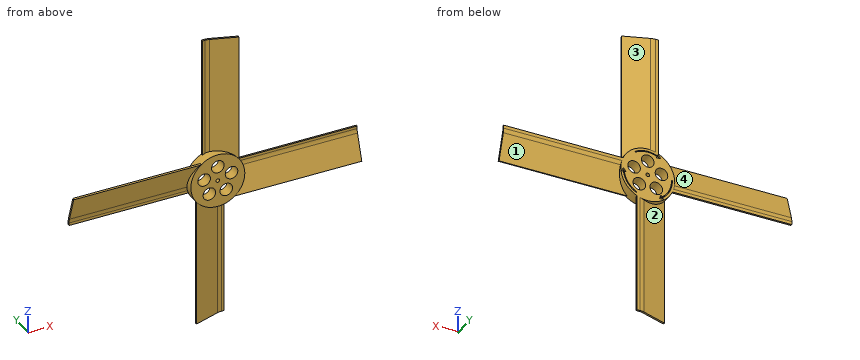
```python
from build123d import *

# Parameters (mm, degrees)
F1_DEPTH  = 80
F2_R      = 7.644408
F4_COUNT  = 4
F5_R      = 15
F6_DEPTH  = 6
F7_R      = 3.5
F7_R_2    = 1
F8_DEPTH  = 25
F10_DEPTH = 1


with BuildPart() as f1:
    # F0 (on Top) → F1 (new body)
    with BuildSketch(Plane.XY):
        Polygon((11.683772, -5.948683), (12, -5), (-3, 0), (-3.316228, -0.948683), align=None)
        Polygon((-3.316228, -0.948683), (-3, 0), (-6, 0), (-6, -0.948683), align=None)
    extrude(amount=-F1_DEPTH)

    # F2
    f2_edges = [f1.edges().sort_by_distance(p)[0] for p in [
        (-3.316228, -0.948683, -40),
        (-3, 0, -40),
    ]]
    fillet(f2_edges, radius=F2_R)



with BuildPart() as f4_1:
    # F4: instance of F1
    add(f1.part.rotate(Axis((0, 13.525062, 0), (0, 1, 0)), 1 * 360 / F4_COUNT))


with BuildPart() as f4_2:
    # F4: instance of F1
    add(f1.part.rotate(Axis((0, 13.525062, 0), (0, 1, 0)), 2 * 360 / F4_COUNT))


with BuildPart() as f4_3:
    # F4: instance of F1
    add(f1.part.rotate(Axis((0, 13.525062, 0), (0, 1, 0)), 3 * 360 / F4_COUNT))


with BuildPart() as f1_1:
    add(f1.part)

    add(f4_1.part)  # F6 merges F4_1

    add(f4_2.part)  # F6 merges F4_2

    add(f4_3.part)  # F6 merges F4_3
    # F5 (on Front) → F6 (join)
    with BuildSketch(Plane.XZ):
        Circle(F5_R)
    extrude(amount=F6_DEPTH)

    # F7 (on face) → F8 (cut)
    with BuildSketch(Plane(origin=(0, 0, 0), x_dir=(-1, 0, 0), z_dir=(0, 1, 0))):
        with Locations((-4.702282, 6.472136)):
            Circle(F7_R)
        with Locations((-7.608452, -2.472136)):
            Circle(F7_R)
        with Locations((0, -8)):
            Circle(F7_R)
        with Locations((7.608452, -2.472136)):
            Circle(F7_R)
        with Locations((4.702282, 6.472136)):
            Circle(F7_R)
        Circle(F7_R_2)
    extrude(amount=-F8_DEPTH, mode=Mode.SUBTRACT)

    # F9 (on face) → F10 (cut)
    with BuildSketch(Plane(origin=(0, 0, 0), x_dir=(-1, 0, 0), z_dir=(0, 1, 0))):
        with BuildLine():
            ThreePointArc((5.158171, -12.103592), (-1.067262, -13.113528), (-7.047458, -11.110221))
            Line((-7.047458, -11.110221), (-7.288358, -11.549476))
            ThreePointArc((-7.288358, -11.549476), (-1.091943, -13.613164), (5.354197, -12.563564))
            Line((5.354197, -12.563564), (5.746248, -13.483508))
            Line((5.746248, -13.483508), (7.096071, -11.549476))
            Line((7.096071, -11.549476), (4.76612, -11.183649))
            Line((4.76612, -11.183649), (5.158171, -12.103592))
        make_face()
        with BuildLine():
            Line((8.803936, 11.71815), (6.454104, 11.920116))
            Line((6.454104, 11.920116), (7.302264, 9.719405))
            Line((7.302264, 9.719405), (7.902933, 10.518903))
            ThreePointArc((7.902933, 10.518903), (11.89028, 5.632489), (13.145463, -0.548167))
            Line((13.145463, -0.548167), (13.646319, -0.537165))
            ThreePointArc((13.646319, -0.537165), (12.335317, 5.860932), (8.203267, 10.918652))
            Line((8.203267, 10.918652), (8.803936, 11.71815))
        make_face()
        with BuildLine():
            Line((-14.550184, 1.765357), (-13.550175, -0.370639))
            Line((-13.550175, -0.370639), (-12.068384, 1.464243))
            Line((-12.068384, 1.464243), (-13.061104, 1.584689))
            ThreePointArc((-13.061104, 1.584689), (-10.823018, 7.48104), (-6.098005, 11.658388))
            Line((-6.098005, 11.658388), (-6.357961, 12.086641))
            ThreePointArc((-6.357961, 12.086641), (-11.243374, 7.752232), (-13.557464, 1.644912))
            Line((-13.557464, 1.644912), (-14.550184, 1.765357))
        make_face()
    extrude(amount=-F10_DEPTH, mode=Mode.SUBTRACT)


with BuildPart() as f11_1:
    # F11: instance of F1
    add(f1_1.part.mirror(Plane.XY))


solid = f11_1.part
```
Check sheet for the modelled part. Datum: model origin and axes. Units: mm. Face numbers are marked on the shaded views. A direction names the side the tool comes from. Give positions to 0.01 mm unless a question says otherwise; leave off trailing zeros. Write each loop counter-clockwise with the first axis right and the second up, starting at its lowest first coordinate (ties: lowest second). Pieces come first, ordered by that corner, then holes.
Item 1: Cross-section at C-C (y = -3.5). Enter the section's corners in (x, z), and give its area (3 significant figures).
Item 2: Gauge pin test, flat ends, axial feed: pin 1 (6.5 mm diameter, centred on x = 7.61, z = 2.47, fed in from -Y); pin 2 (0.8 mm diameter, centred on x = 54, y = -0.5, fed in from +Z); pin 3 (0.5 mm diameter, centred on x = -40, y = -0.5, fed in from -Z); pin 4 (10 mm diameter, centred on x = 10.5, z = 18.5, fed in from +Y). Record the tip position at first contact, or that the pin passes through.
Item 3: Access from +Z, -Z, +X, -X, +Y, -Y to the whole of each face (thin tool, end or side, straight path). Record for the marked faces 1, 2, 3 and 4.
Item 4: Scan lines: L1, parallel to Z at x = 0, y = -1.9; L2, parallel to Z at x = 0, y = -3.9; L3, parallel to X at y = -2.5, z = 8.5. Record each from-to range of solid material in increasing order.
Item 5: Cross-section at B-B (x = -22.5). Enter the section's corners in (y, z), and give its area (3 significant figures).
Item 6: Cross-section at A-A (z = 57). Enter the section's corners in (x, y), and give its area (3 significant figures).
Report:
1. outline: (-80, 4.34) - (-14.36, 4.34) arc R15 ccw to (-7.5, -12.99) - (-7.5, -80) - (-4.34, -80) - (-4.34, -14.36) arc R15 ccw to (12.99, -7.5) - (80, -7.5) - (80, -4.34) - (14.36, -4.34) arc R15 ccw to (7.5, 12.99) - (7.5, 80) - (4.34, 80) - (4.34, 14.36) arc R15 ccw to (-12.99, 7.5) - (-80, 7.5) - close; hole circle Ø7 at (-7.61, 2.47); hole circle Ø7 at (-4.7, -6.47); hole circle Ø7 at (0, 8); hole circle Ø2 at (0, 0); hole circle Ø7 at (4.7, -6.47); hole circle Ø7 at (7.61, 2.47)
1. area: 1,350 mm2
2. pin 1: passes through
2. pin 2: stops at z = 6
2. pin 3: stops at z = -6
2. pin 4: stops at y = -2.83
3. face 1: -Z, +X, +Y
3. face 2: -Z, -X, +Y
3. face 3: +Z, +X, +Y
3. face 4: +Z, -X, +Y
4. L1: z = -80 to -1, 1 to 4.5, 11.5 to 80
4. L2: z = -15 to -1, 1 to 4.5, 11.5 to 15
4. L3: x = -12.36 to -3.46, 3.46 to 12.36
5. outline: (-5.95, 11.68) - (-1.34, -2.14) arc R7.64 cw to (-0.95, -4.56) - (-0.95, -6) - (0, -6) - (0, -4.24) arc R7.64 ccw to (-0.39, -1.82) - (-5, 12) - close
5. area: 18.5 mm2
6. outline: (-6, -0.95) - (-4.56, -0.95) arc R7.64 cw to (-2.14, -1.34) - (11.68, -5.95) - (12, -5) - (-1.82, -0.39) arc R7.64 ccw to (-4.24, 0) - (-6, 0) - close
6. area: 18.5 mm2
